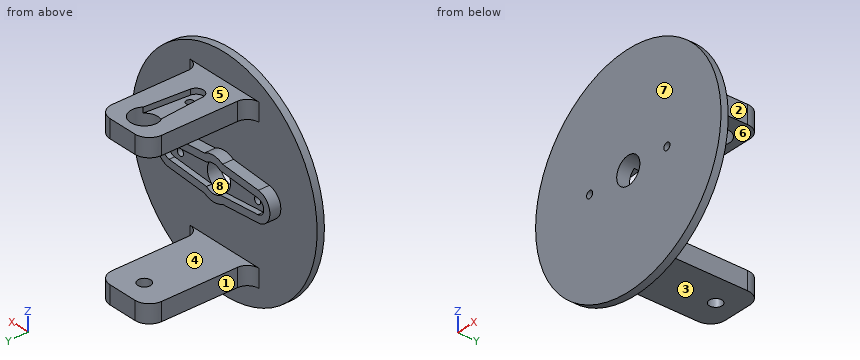
Autodesk Inventor part; units mm, degrees
ref_plane "YZ Plane" through (0, 0, 0) normal (1, 0, 0) x (0, 1, 0)
ref_plane "XZ Plane" through (0, 0, 0) normal (0, 1, 0) x (-1, 0, 0)
ref_plane "XY Plane" through (0, 0, 0) normal (0, 0, 1) x (1, 0, 0)
sketch "スケッチ1" plane through (0, 0, 0) normal (0, 1, 0) x (-1, 0, 0)
  circle A0 centre (0, 0) radius 30
  line L0 (0, -50.5872) -> (0, 52.7432)
  line L1 (-2.25, -3) -> (-14.3614, -2.0436)
  line L2 (47.5195, 0) -> (-63.2606, 0)
  line L3 (-2.25, 3) -> (-14.3614, 2.0436)
  arc A1 (-14.3614, 2.0436) -> (-14.3614, -2.0436) centre (-14.2, 0) ccw
  line L4 (2.25, -3) -> (14.3614, -2.0436)
  line L5 (2.25, 3) -> (14.3614, 2.0436)
  arc A2 (14.3614, -2.0436) -> (14.3614, 2.0436) centre (14.2, 0) ccw
  arc A3 (-2.25, -3) -> (2.25, -3) centre (0, 0) ccw
  arc A4 (2.25, 3) -> (-2.25, 3) centre (0, 0) ccw
  circle A5 centre (-12.5, 0) radius 1
  circle A6 centre (12.5, 0) radius 1
  line L6 (14.5188, -4.0374) -> (2.9201, -4.9533)
  arc A7 (-2.9201, -4.9533) -> (2.9201, -4.9533) centre (0, 0) ccw
  line L7 (-2.9201, -4.9533) -> (-14.5188, -4.0374)
  arc A8 (-14.5188, 4.0374) -> (-14.5188, -4.0374) centre (-14.2, 0) ccw
  line L8 (-14.5188, 4.0374) -> (-2.9201, 4.9533)
  arc A9 (2.9201, 4.9533) -> (-2.9201, 4.9533) centre (0, 0) ccw
  line L9 (2.9201, 4.9533) -> (14.5188, 4.0374)
  arc A10 (14.5188, -4.0374) -> (14.5188, 4.0374) centre (14.2, 0) ccw
  arc A11 (2.25, -3) -> (2.25, 3) centre (0, 0) ccw
  arc A12 (-2.25, 3) -> (-2.25, -3) centre (0, 0) ccw
  dimension "d0" = 60
  dimension "d1" = 14.2
  dimension "d2" = 2.05
  dimension "d3" = 6
  dimension "d5" = 12.5
  dimension "d6" = 2
  dimension "d7" = 2
  dimension "d10" = 3.75
extrude "押し出し1" add sketch "スケッチ1" along normal blind 2 contours L2 A10 L9 A9 L0 A0 | A0 L0 A7 L6 A10 L2 | L0 A9 L8 A8 L2 A0 | A0 L2 A8 L7 A7 L0
extrude "押し出し2" add sketch "スケッチ1" along normal blind 5 contours A10 L6 A7 L0 A3 L4 A2 L2 | L2 A2 L5 A4 L0 A9 L9 A10 | L0 A4 L3 A1 L2 A8 L8 A9 | A7 L7 A8 L2 A1 L1 A3 L0
extrude "押し出し3" add sketch "スケッチ1" along normal blind 3.5 contours A2 L4 A11 L2 A6 | L2 A6 A11 L5 A2 | A1 L3 A12 L2 A5 | L2 A5 A12 L1 A1
sketch "スケッチ2" plane through (0, 2, 0) normal (0, 1, 0) x (1, 0, 0)
  line L0 (0, 57.7571) -> (0, -77.3728)
  line L1 (-74.0829, 0) -> (96.0409, 0)
  line L2 (-8, 18) -> (8, 18)
  line L3 (8, 18) -> (8, 23)
  line L4 (8, 23) -> (-8, 23)
  line L5 (-8, 23) -> (-8, 18)
  line L6 (-8, -18) -> (8, -18)
  line L7 (8, -18) -> (8, -23)
  line L8 (8, -23) -> (-8, -23)
  line L9 (-8, -23) -> (-8, -18)
  point P0 (0, 0)
  dimension "d15" = 36
  dimension "d16" = 16
  dimension "d17" = 5
extrude "押し出し4" add sketch "スケッチ2" along normal blind 28
sketch "スケッチ4" plane through (-8, 2, 23) normal (0, 0, 1) x (1, 0, 0)
  line L0 (0, 28) -> (16, 28)
  line L1 (8, 28) -> (8, 0)
  line L2 (38, 0) -> (-22, 0)
  circle A0 centre (8, 22) radius 3.75
  arc A1 (5.9564, 7.6386) -> (10.0436, 7.6386) centre (8, 7.8) ccw
  line L3 (5, 19.75) -> (5.9564, 7.6386)
  line L4 (11, 19.75) -> (10.0436, 7.6386)
  circle A2 centre (8, 9.5) radius 1
  point P0 (8, -2)
  dimension "d20" = 14.2
  dimension "d21" = 2
  dimension "d22" = 6
  dimension "d23" = 7.5
  dimension "d24" = 22
  dimension "d25" = 2.05
  dimension "d26" = 12.5
extrude "押し出し5" cut sketch "スケッチ4" against normal up to surface (5 mm away) contours A0 L1 | L1 A0 | A2 L1 | L1 A2
extrude "押し出し6" cut sketch "スケッチ4" against normal blind 1.5 contours A0 L4 A1 L1 A2 | L1 A2 A1 L3 A0
sketch "スケッチ5" plane through (8, 2, -23) normal (0, 0, -1) x (-1, 0, 0)
  line L0 (16, 28) -> (0, 28)
  line L1 (8, 28) -> (8, 0)
  line L2 (38, 0) -> (-22, 0)
  circle A0 centre (8, 22) radius 1.75
  circle A1 centre (8, 22) radius 3.75
  point P0 (8, -2)
  dimension "d31" = 3.5
extrude "押し出し7" cut sketch "スケッチ5" against normal up to surface (5 mm away) contours A0 L1 | L1 A0
fillet "フィレット1" radius 3.2 4 edges at (8, 2, -20.5) (8, 2, 20.5) (-8, 2, -20.5) (-8, 2, 20.5)
fillet "フィレット2" radius 4 4 edges at (-8, 30, -20.5) (8, 30, -20.5) (-8, 30, 20.5) (8, 30, 20.5)
properties part number "axis1"
Design review of the part built by this model. Coordinates are the model's own, in mm. Face numbers are marked on the shaded views. A direction names the side the tool comes from. Coordinates: 2 decimals unless noted, no trailing zeros. Write each loop counter-clockwise with the first axis right and the second up, starting at its lowest first coordinate (ties: lowest second). Pieces come first, ordered by that corner, then holes.
1) Machinability: for the marked faces 1, 2, 3 and 4, which of the approach directions +Z, -Z, +X, -X, +Y, -Y give a long, thin tool a straight path to every point of the face, cutting with its end or side? Answer none if there is none.
2) Mouldability with a two-part tool opening along Z and no side actions: class the marked faces 5, 6, 7 and 8 as +Z half, -Z half, draft (parallel to the pull), parting line (faces both ways), or undercut.
3) Add section D-D (y = 6.5). Write out the cut boundary in (x, z), plus the area to 3 significant figures.
4) Add section B-B (y = 24). Write out the cut boundary in (x, z).
5) To check wall thickness, follow L1, parallel to X at y = 1.3, z = 0; L2, parallel to Z at x = -1, y = 5.75; L3, parallel to X at y = 2.5, z = 0. State the ranges of each line that lie inside material, in increasing order.
6) Add section C-C (z = 0). Write out the cut boundary in (x, y), plus the area to 4 significant figures.
7) Insertion check: pin 1 (6.5 mm diameter, centred on x = -5.5, y = 16.5, fed in from +Z); pin 2 (4 mm diameter, centred on y = 20.5, z = 19.5, fed in from +X); pin 3 (3.5 mm diameter, centred on x = -4, z = -2, fed in from +Y). Each pin has a flat end and moves straight along its axis. Give the tip position at first contact, or say it passes through.
8) Add section A-A (x = 0). State how many separate pieces and enclosed holes the cut face has, plus the area to 3 significant figures.
Check result:
1. face 1: +Z, -Z, -X, +Y
1. face 2: +Z, -Z, +X, +Y
1. face 3: -Z, +X, -X, +Y
1. face 4: +X, -X, +Y
2. face 5: +Z half
2. face 6: undercut
2. face 7: draft
2. face 8: undercut
3. outline: (-8, -23) - (8, -23) - (8, -18) - (-8, -18) - close; (-8, 18) - (8, 18) - (8, 23) - (-8, 23) - close
3. area: 160 mm2
4. outline: (-8, -23) - (-1.75, -23) - (-1.75, -18) - (-8, -18) - close; (-8, 18) - (-3.75, 18) - (-3.75, 23) - (-8, 23) - close; (1.75, -23) - (8, -23) - (8, -18) - (1.75, -18) - close; (3.75, 18) - (8, 18) - (8, 23) - (3.75, 23) - close
5. L1: x = -30 to -13.5, -11.5 to -3.75, 3.75 to 11.5, 13.5 to 30
5. L2: z = -23 to -18, 18 to 23
5. L3: x = -18.25 to -13.5, -11.5 to -3.75, 3.75 to 11.5, 13.5 to 18.25
6. outline: (-30, 0) - (-13.5, 0) - (-13.5, 3.5) - (-16.25, 3.5) - (-16.25, 5) - (-18.25, 5) - (-18.25, 2) - (-30, 2) - close; (-11.5, 0) - (-3.75, 0) - (-3.75, 3.5) - (-11.5, 3.5) - close; (3.75, 0) - (11.5, 0) - (11.5, 3.5) - (3.75, 3.5) - close; (13.5, 0) - (30, 0) - (30, 2) - (18.25, 2) - (18.25, 5) - (16.25, 5) - (16.25, 3.5) - (13.5, 3.5) - close
6. area: 140.5 mm2
7. pin 1: stops at z = 23
7. pin 2: stops at x = 8
7. pin 3: stops at y = 5
8. separate pieces: 5
8. enclosed holes: 0
8. area: 316 mm2
